from build123d import *

# Parameters (mm, degrees)
F2_R     = 2.261012
F2_R_2   = 15.5
F3_DEPTH = 12
F5_DEPTH = 7.1


with BuildPart() as f3:
    # F2 (on offset) → F3 (new body)
    with BuildSketch(Plane.XY.offset(19)):
        with BuildLine():
            ThreePointArc((-22, 2), (-23.464466, -1.535534), (-27, -3))
            Line((-27, -3), (-66.61081, -3))
            ThreePointArc((-66.61081, -3), (0, -54), (66.61081, -3))
            Line((66.61081, -3), (27, -3))
            ThreePointArc((27, -3), (23.464466, -1.535534), (22, 2))
            Line((22, 2), (22, 30.368569))
            ThreePointArc((22, 30.368569), (0, 37.5), (-22, 30.368569))
            Line((-22, 30.368569), (-22, 2))
        make_face()
        with Locations((-15, -25)):
            Circle(F2_R, mode=Mode.SUBTRACT)
        with Locations((0, -30)):
            Circle(F2_R, mode=Mode.SUBTRACT)
        with Locations((15, -25)):
            Circle(F2_R, mode=Mode.SUBTRACT)
        with Locations((-15, 25)):
            Circle(F2_R, mode=Mode.SUBTRACT)
        Circle(F2_R_2, mode=Mode.SUBTRACT)
        with Locations((15, 25)):
            Circle(F2_R, mode=Mode.SUBTRACT)
        with Locations((0, 30)):
            Circle(F2_R, mode=Mode.SUBTRACT)
    extrude(amount=F3_DEPTH)

    # F4 (on offset) → F5 (cut)
    with BuildSketch(Plane.XY.offset(19)):
        with BuildLine():
            Line((-3, 0), (-3, -20))
            ThreePointArc((-3, -20), (0, -23), (3, -20))
            Line((3, -20), (3, 0))
            Line((3, 0), (3, 20))
            ThreePointArc((3, 20), (0, 23), (-3, 20))
            Line((-3, 20), (-3, 0))
        make_face()
    extrude(amount=F5_DEPTH, mode=Mode.SUBTRACT)


solid = f3.part
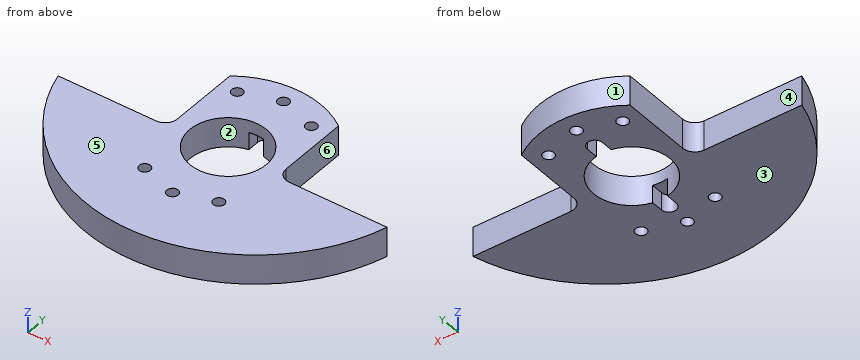
The model under review builds one solid part; all positions refer to its coordinate system, in mm. Face numbers are marked on the shaded views. A direction names the side the tool comes from. Round coordinates to 2 decimals unless told otherwise and drop trailing zeros. Loops run counter-clockwise (first coordinate to the right, second up) from the corner with the lowest first, then second, coordinate; pieces in that order, holes last. Notation, with made-up numbers: M 83.25,-34 L 114.25,-34 A17 cw 114.25,-23 Z; hole C -35,-6.75 d3. An arc over 180 degrees is marked long. Answer as CSV lines item,"result".
1. We need section D-D (y = -12). Give the boundary of the cut face in (x, z).
Outcome:
outline,"M -63.5,19 L -9.81,19 L -9.81,31 L -63.5,31 Z; M 9.81,19 L 63.5,19 L 63.5,31 L 9.81,31 Z"
2. Insertion check: pin 1 Ø3.5 at (x, y) = (-15, 25) entering from -Z; pin 2 Ø4 at (x, z) = (-46, 27) entering from +Y; pin 3 Ø1 at (x, z) = (7, 22.5) entering from +Y; pin 4 Ø4 at (y, z) = (-17.5, 20.5) entering from -X. Each pin has a flat end and moves straight along its axis. Give the tip position at first contact, or say it passes through.
Outcome:
pin 1,"passes through"
pin 2,"stops at y = -3"
pin 3,"stops at y = 36.93"
pin 4,"stops at x = -61.89"
3. We need section B-B (y = 25). Give the boundary of the cut face in (x, z), plus the area to 3 significant figures.
Outcome:
outline,"M -22,19 L -17.26,19 L -17.26,31 L -22,31 Z; M -12.74,19 L 12.74,19 L 12.74,31 L -12.74,31 Z; M 17.26,19 L 22,19 L 22,31 L 17.26,31 Z"
area,"419 mm2"
4. We need section C-C (z = 21.75). Give the boundary of the cut face in (x, y), plus the area to 3 significant figures.
Outcome:
outline,"M -66.61,-3 A69 ccw 66.61,-3 L 27,-3 A5 cw 22,2 L 22,30.37 A37.5 ccw -22,30.37 L -22,2 A5 cw -27,-3 Z; hole C -15,-25 d4.52; hole C -15,25 d4.52; hole M -3,-20 A3 ccw 3,-20 L 3,-15.21 A15.5 ccw 3,15.21 L 3,20 A3 ccw -3,20 L -3,15.21 A15.5 ccw -3,-15.21 Z; hole C 0,-30 d4.52; hole C 0,30 d4.52; hole C 15,-25 d4.52; hole C 15,25 d4.52"
area,"5,780 mm2"
5. Draft analysis for pull direction X (two halves, no side actions). For the marked faces 1, 2 and 3, state which applies: pulls with the +X half, pulls with the -X half, needs draft (parallel to the pull), parting line crosses it, or undercut.
Outcome:
face 1,"parting line crosses it"
face 2,"undercut"
face 3,"needs draft"
6. To check wall thickness, follow L1, parallel to Y at x = 0, z = 27; L2, parallel to Y at x = 0, z = 23.5; L3, parallel to X at y = 15.5, z = 20. State the ranges of each line that lie inside material, in increasing order. Write a range as [from, to].
Outcome:
L1,"y = [-54, -32.26], [-27.74, -15.5], [15.5, 27.74], [32.26, 37.5]"
L2,"y = [-54, -32.26], [-27.74, -23], [23, 27.74], [32.26, 37.5]"
L3,"x = [-22, -3], [3, 22]"
7. We need section A-A (x = 0). Give the boundary of the cut face in (y, z), plus the area to 3 significant figures.
Outcome:
outline,"M -54,19 L -32.26,19 L -32.26,31 L -54,31 Z; M -27.74,19 L -23,19 L -23,26.1 L -15.5,26.1 L -15.5,31 L -27.74,31 Z; M 15.5,26.1 L 23,26.1 L 23,19 L 27.74,19 L 27.74,31 L 15.5,31 Z; M 32.26,19 L 37.5,19 L 37.5,31 L 32.26,31 Z"
area,"511 mm2"
8. For the marked faces 4, 5 and 6, list the 3-axis set-ups (+Z, -Z, +X, -X, +Y, -Y) from which the entire face can be reached by the end or side of a thin tool; tool diameter is ignored.
Outcome:
face 4,"+Z, -Z, -X, +Y"
face 5,"+Z, +X, -X, +Y, -Y"
face 6,"+Z, -Z, +X, +Y"
